Verification items for the finished model (mm, model axes). Coordinates: 2 decimals unless noted, no trailing zeros. Write each loop counter-clockwise with the first axis right and the second up, starting at its lowest first coordinate (ties: lowest second). Pieces come first, ordered by that corner, then holes. Notation, with made-up numbers: (2.25, 81.5) -> (17.25, 81.5) arc R19 cw to (17.25, 89.5) -> close; hole circle Ø10 at (88.25, 78.25). An arc over 180 degrees is marked (long way). Answer in a Markdown table with one row per item.
```python
from build123d import *

# Parameters (mm, degrees)
F0_R     = 50.8
F0_W     = 3.175
F0_H     = 6.35
F0_R_2   = 1.4732
F0_R_3   = 1.524
F1_DEPTH = 3.175


# Not quite as in the source:
# - a length typed as a fraction of an inch, garbled in the dataset ("3 / 203.2 mm" for 3/8 in), is restored


with BuildPart() as f1:
    # F0 (on Top) → F1 (new body)
    with BuildSketch(Plane.XY):
        Circle(F0_R)
        with Locations((-11.43, -12.7)):
            Rectangle(F0_W, F0_H, mode=Mode.SUBTRACT)
        with Locations((0, -7)):
            Circle(F0_R_2, mode=Mode.SUBTRACT)
        with Locations((-11.43, 0)):
            Circle(F0_R_3, mode=Mode.SUBTRACT)
        with Locations((-7, 0)):
            Circle(F0_R_2, mode=Mode.SUBTRACT)
        with Locations((11.43, -12.7)):
            Rectangle(F0_W, F0_H, mode=Mode.SUBTRACT)
        with Locations((7, 0)):
            Circle(F0_R_2, mode=Mode.SUBTRACT)
        with Locations((11.43, 0)):
            Circle(F0_R_3, mode=Mode.SUBTRACT)
        with Locations((0, 7)):
            Circle(F0_R_2, mode=Mode.SUBTRACT)
        with Locations((-11.43, 12.7)):
            Rectangle(F0_W, F0_H, mode=Mode.SUBTRACT)
        with Locations((11.43, 12.7)):
            Rectangle(F0_W, F0_H, mode=Mode.SUBTRACT)
    extrude(amount=F1_DEPTH)


solid = f1.part
```
1. Section check D-D, the plane x = 19.5. Record the boundary of the cut face in (y, z) (3 decimals).
Geometry says:
| item | result |
|---|---|
| outline | (-46.908, 0) -> (46.908, 0) -> (46.908, 3.175) -> (-46.908, 3.175) -> close |
2. Section check A-A, the plane z = 2.45. State how many separate pieces and enclosed holes the cut face has, plus the area to 3 significant figures.
Geometry says:
| item | result |
|---|---|
| separate pieces | 1 |
| enclosed holes | 10 |
| area | 7,980 mm^2 |
3. Section check B-B, the plane y = -7. Record the boundary of the cut face in (x, z) (3 decimals).
Geometry says:
| item | result |
|---|---|
| outline | (-50.315, 0) -> (-1.473, 0) -> (-1.473, 3.175) -> (-50.315, 3.175) -> close; (1.473, 0) -> (50.315, 0) -> (50.315, 3.175) -> (1.473, 3.175) -> close |
4. Mould release check, pull along Y, two halves, no side actions. Record for faces 1 (the flat face through (9.842, 13, 2)), 2 (the flat face through (-1, 1, 0)), 3 (the cylindrical face through (5.53, 0.06, 1.57)), 4 (the cylindrical face through (-11.012, -49.592, 1.565)): released by +Y, released by -Y, zero draft, split by the parting line, or undercut.
Geometry says:
| item | result |
|---|---|
| face 1 | undercut |
| face 2 | zero draft |
| face 3 | undercut |
| face 4 | split by the parting line |
5. Depth check by flat-ended pin: P1, Ø1, axis at y = 12, z = 2, coming from the -X side; P2, Ø1, axis at y = -11.5, z = 1.5, coming from the -X side; P3, Ø1.8, axis at x = -7, y = 0, coming from the -Z side; P4, Ø1.5, axis at y = 7, z = 0.5, coming from the +X side. Enter the tip coordinate at first touch or a pass-through.
Geometry says:
| item | result |
|---|---|
| P1 | x = -49.48 |
| P2 | x = -49.59 |
| P3 | through |
| P4 | x = 50.41 |
6. Thickness scan on line 1 (Y direction, x = 0, z = 1.55); line 2 (Y direction, x = -7, z = 2.3); line 3 (X direction, y = 2.5, z = 1.2). Record the ranges inside material, lowest first. Write a range as from..to.
Geometry says:
| item | result |
|---|---|
| line 1 | -50.8..-8.47, -5.53..5.53, 8.47..50.8 |
| line 2 | -50.32..-1.47, 1.47..50.32 |
| line 3 | -50.74..50.74 |
